Can you work these out from the model? Positions are in its coordinate system, mm. Give positions to 0.01 mm unless a question says otherwise; leave off trailing zeros. Order: outer loops, then holes, each group sorted by start corner. A loop starts at its lowest first (then second) coordinate and runs counter-clockwise, first axis right, second up. Notation, with made-up numbers: M 28.25,-12.5 L 69.25,-12.5 A4 cw 69.25,-6.5 Z; hole C 18,-38 d1. An arc over 180 degrees is marked long. Use a Markdown table: item, result. Add a question column.
Autodesk Inventor part; units mm, degrees
ref_plane "YZ Plane" through (0, 0, 0) normal (1, 0, 0) x (0, 1, 0)
ref_plane "XZ Plane" through (0, 0, 0) normal (0, 1, 0) x (-1, 0, 0)
ref_plane "XY Plane" through (0, 0, 0) normal (0, 0, 1) x (1, 0, 0)
sketch "Sketch1" plane through (0, 0, 0) normal (0, 1, 0) x (-1, 0, 0)
  line L0 (30, 275) -> (0, 275)
  line L1 (0, 275) -> (0, -275)
  line L2 (0, -275) -> (30, -275)
  line L3 (30, -275) -> (30, 275)
  line L4 (539.12, 64.1138) -> (150.2089, -324.7926)
  arc A0 (539.12, 64.1138) -> (30, 275) centre (30, -445) ccw
  arc A1 (150.2089, -324.7926) -> (30, -275) centre (30, -445) ccw
  line L5 (0, 255) -> (30, 255)
  line L6 (0, -255) -> (30, -255)
  arc A2 (524.9778, 49.9717) -> (30, 255) centre (21.7353, -464.9526) ccw
  arc A3 (164.3511, -310.6505) -> (30, -255) centre (38.3697, -424.7938) ccw
  point P0 (0, 0)
  point P1 (0, 0)
  dimension "d0" = 30
  dimension "d1" = 550
  dimension "d4" = 550
  dimension "d8" = 539.12
  dimension "d9" = 720
  dimension "d10" = 170
  dimension "d19" = 20
  dimension "d20" = 20
  dimension "d21" = 20
  dimension "d22" = 20
  dimension "d26" = 170
  dimension "d27" = 720
extrude "Extrusion1" add sketch "Sketch1" along normal blind 3 contours A0 L4 A2 L3 | A2 L4 A3 L3 | A3 L4 A1 L3
extrude "Extrusion2" add sketch "Sketch1" along normal blind 3.1 contours A0 L4 A2 L3 | A3 L4 A1 L3
equation "\"d1\" = track_width"
equation "\"d4\" = d1"
equation "\"d19\" = curb_width"
equation "\"d20\" = curb_width"
equation "\"d21\" = curb_width"
equation "\"d22\" = curb_width"
equation "\"d26\" = d10"
equation "\"d27\" = d9"
equation "\"d6\" = track_height"
equation "\"d24\" = track_height + curb_height"
properties part number "curve_left"
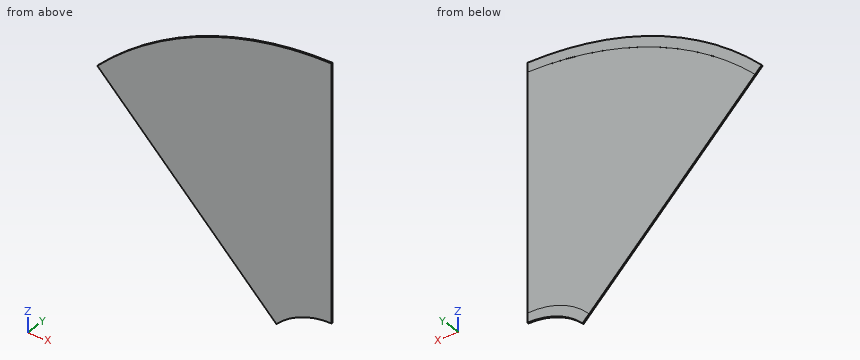
1. If we section it at B-B, the plane x = -130: List the corners of the cut face in (y, z) for me.
2. If we section it at C-C, the plane z = 222: List the corners of the cut face in (x, y) for me, then the cut area to 3 significant figures.
3. If we section it at A-A, the plane y = 1: List the corners of the cut face in (x, z) for me, then the cut area to 3 significant figures.
4. I need wall thicknesses on L1, parallel to Y at x = -349.5, z = -85; L2, parallel to X at y = 1.4, z = -135.5; L3, parallel to Z at x = -405, y = 2.3. Which ranges of each line are inside material? Lowest first, please. Write a range as [from, to].
5. If we section it at D-D, the plane x = -70.5: List the corners of the cut face in (y, z) for me, then the cut area to 3 significant figures.
6. Will this pin go through, and if not, where does the flat tip stop? pin 1 (1 mm diameter, centred on x = -138, z = -168, fed in from +Y).
Geometry results:
| question | item | result |
|---|---|---|
| 1 | outline | M 0,-307.52 L 3.1,-307.52 L 3.1,-281.6 L 3,-281.6 L 3,246.86 L 3.1,246.86 L 3.1,268.02 L 0,268.02 Z |
| 2 | outline | M -301.13,0 L -30,0 L -30,3 L -237.37,3 L -237.37,3.1 L -301.13,3.1 Z |
| 2 | area | 820 mm^2 |
| 3 | outline | M -539.12,64.11 L -150.21,-324.79 A170 cw -30,-275 L -30,275 A720 ccw Z |
| 3 | area | 192,000 mm^2 |
| 4 | L1 | y = [0, 3] |
| 4 | L2 | x = [-339.5, -30] |
| 4 | L3 | z = [-70, 169.63] |
| 5 | outline | M 0,-279.89 L 3.1,-279.89 L 3.1,-257.86 L 3,-257.86 L 3,253.39 L 3.1,253.39 L 3.1,273.86 L 0,273.86 Z |
| 5 | area | 1,670 mm^2 |
| 6 | pin 1 | stops at y = 3 |
